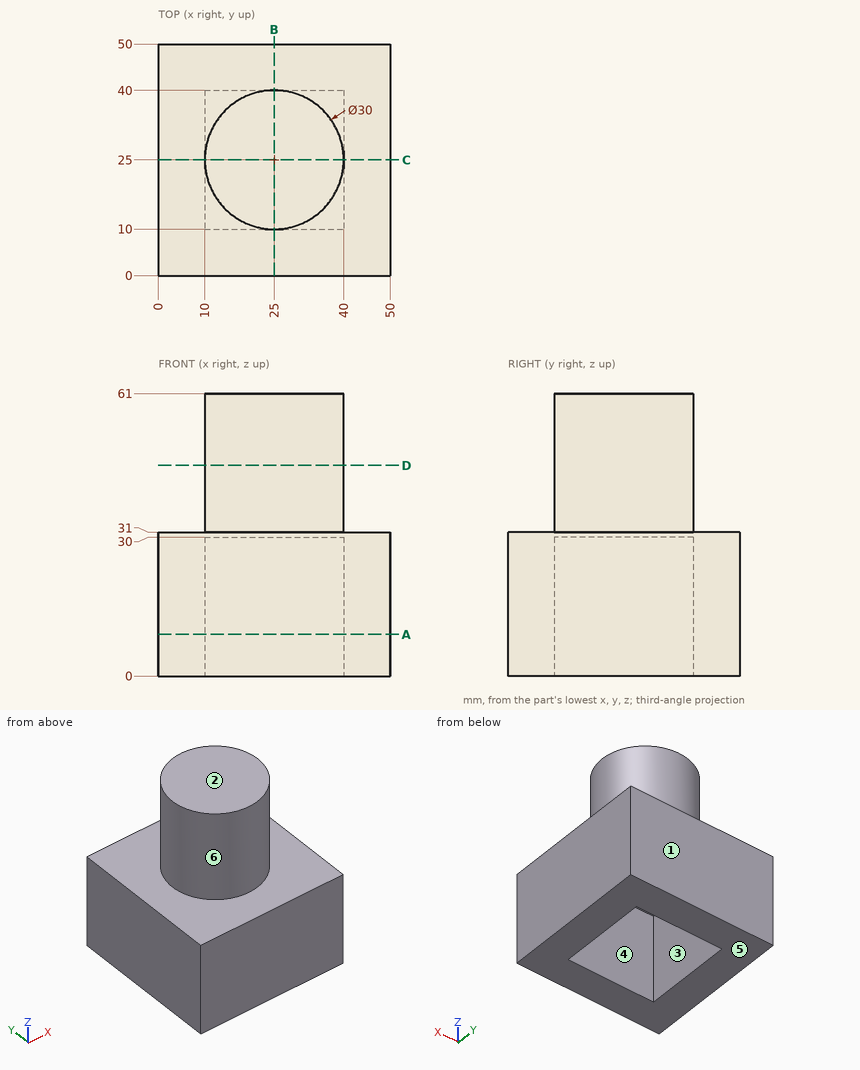
Job drawing, mm, ordinate dimensions from the low corner. One solid piece. A direction names the side the tool comes from. Give positions to 0.01 mm unless a question says otherwise; leave off trailing zeros. Write each loop counter-clockwise with the first axis right and the second up, starting at its lowest first coordinate (ties: lowest second). Pieces come first, ordered by that corner, then holes. Notation, with made-up numbers: M 56,24.5 L 96,24.5 A33 ccw 96,55.5 Z; hole C 11,-4 d2. An arc over 180 degrees is marked long. Put each result on its own line as item: value. Start each with the question number.
(1) Probe L1, parallel to Y at x = 10.5, z = 26.5; L2, parallel to Z at x = 4.5, y = 5. List the from-to ranges inside material, lowest first.
(2) Band-saw the part on B-B, the plane x = 25. Write the cut outline in (y, z), and give its area (3 significant figures).
(3) Band-saw the part on D-D, the plane z = 45.5. Write the cut outline in (x, y).
(4) Mould opens along Y. For the marked faces 1, 2 and 3 say: +Y half, -Y half, draft (parallel to the pull), parting line (faces both ways), or undercut.
(5) Band-saw the part on A-A, the plane z = 9. Write the cut outline in (x, y).
(6) Flat gauge pins, fed straight in: pin 1 Ø1.5 at (y, z) = (33.5, 46) entering from -X; pin 2 Ø6 at (x, y) = (10.5, 9.5) entering from +Z; pin 3 Ø10 at (x, z) = (42.5, 47) entering from -Y. Where does each tip first touch, or does it go through?
(7) Which spindle directions (+Z, -Z, +X, -X, +Y, -Y) get a long thin tool onto all of the face, cutting with end or side? Do the marked faces 4, 5 and 6. Say none if no direction does.
Response values:
1. L1: y = 0 to 10, 40 to 50
1. L2: z = 0 to 31
2. outline: M 0,0 L 10,0 L 10,30 L 40,30 L 40,0 L 50,0 L 50,31 L 40,31 L 40,61 L 10,61 L 10,31 L 0,31 Z
2. area: 1,550 mm2
3. outline: C 25,25 d30
4. face 1: +Y half
4. face 2: draft
4. face 3: undercut
5. outline: M 0,0 L 50,0 L 50,50 L 0,50 Z; hole M 10,10 L 40,10 L 40,40 L 10,40 Z
6. pin 1: stops at x = 12.16
6. pin 2: stops at z = 31
6. pin 3: stops at y = 16.71
7. face 4: -Z
7. face 5: -Z, +X, -X, +Y, -Y
7. face 6: +Z
